Build history of the part. All positions in model axes, mm. A direction names the side the tool comes from. Round coordinates to 2 decimals unless told otherwise and drop trailing zeros. Write each loop counter-clockwise with the first axis right and the second up, starting at its lowest first coordinate (ties: lowest second). Pieces come first, ordered by that corner, then holes. Notation, with made-up numbers: M 74.25,36 L 102.25,36 A18 ccw 102.25,65 Z; hole C 36.5,50 d9. An arc over 180 degrees is marked long. Use a Markdown table: item, result.
from build123d import *

# Parameters (mm, degrees)
F2_W     = 50
F2_H     = 55
F3_DEPTH = 30
F4_W     = 49
F4_H     = 20.1
F5_DEPTH = 50.001
F0_R     = 2.85
F6_DEPTH = 4.9
F0_W     = 7
F0_H     = 6.6
F7_DEPTH = 15
F8_START = 25
F1_W     = 40
F1_H     = 45
F8_DEPTH = 25


# Not quite as in the source:
# - a feature names something its author has since deleted; it is built from what else it names


with BuildPart() as f3:
    # F2 (on Top) → F3 (new body)
    with BuildSketch(Plane.XY):
        with Locations((-48.7460665315, -28.1598071134)):
            Rectangle(F2_W, F2_H)
    extrude(amount=F3_DEPTH)

    # F4 (on face) → F5 (cut, through all)
    with BuildSketch(Plane.YZ.offset(-23.7460665315)):
        with Locations((-27.83, 14.95)):
            Rectangle(F4_W, F4_H)
    extrude(amount=-F5_DEPTH, mode=Mode.SUBTRACT)

    # F0 (on Top) → F6 (cut, through all)
    with BuildSketch(Plane.XY):
        with Locations((-36.0460665315, -28.1598071134)):
            Circle(F0_R)
        with Locations((-61.4460665315, -28.1598071134)):
            Circle(F0_R)
    extrude(amount=F6_DEPTH, mode=Mode.SUBTRACT)

    # F0 (on Top) → F7 (join)
    with BuildSketch(Plane.XY):
        with Locations((-43.6801504195, -28.1598071134)):
            Rectangle(F0_W, F0_H)
    extrude(amount=F7_DEPTH)

    # F1 (on Top) → F8 (cut)
    with BuildSketch(Plane.XY.offset(F8_START)):
        with Locations((-48.7460665315, -27.7248071134)):
            Rectangle(F1_W, F1_H)
    extrude(amount=F8_DEPTH, mode=Mode.SUBTRACT)


solid = f3.part
Q1. Cut at C-C on x = -70. Give the cut face in (y, z), and give its area (3 significant figures).
Response values:
| item | result |
|---|---|
| outline | M -55.66,0 L -0.66,0 L -0.66,30 L -55.66,30 Z; hole M -52.33,4.9 L -3.33,4.9 L -3.33,25 L -52.33,25 Z |
| area | 665 mm2 |
Q2. Cut at D-D on x = -51.5. Give the cut face in (y, z), and give its area (3 significant figures).
Response values:
| item | result |
|---|---|
| outline | M -55.66,0 L -0.66,0 L -0.66,30 L -5.22,30 L -5.22,25 L -3.33,25 L -3.33,4.9 L -52.33,4.9 L -52.33,25 L -50.22,25 L -50.22,30 L -55.66,30 Z |
| area | 440 mm2 |
Q3. Drop flat-ended pins along their axis: P1, Ø2, axis at y = -28, z = 9.5, coming from the +X side; P2, Ø2, axis at x = -44.5, y = -28, coming from the +Z side; P3, Ø5.5, axis at y = -28, z = 9.5, coming from the -X side. Give the stop position or say it passes through.
Response values:
| item | result |
|---|---|
| P1 | stops at x = -40.18 |
| P2 | stops at z = 15 |
| P3 | stops at x = -47.18 |
Q4. Two-plate mould, pull along Y, no slides. Class faces 1 (the flat face through (-27, -28, 30)), 2 (the flat face through (-49, -55.66, 15)), 3 (the flat face through (-44, -28, 15)): +Y half, -Y half, draft (parallel to the pull), parting line (faces both ways), or undercut.
Response values:
| item | result |
|---|---|
| face 1 | draft |
| face 2 | -Y half |
| face 3 | undercut |
Q5. Cut at A-A on y = -18.5. Give the cut face in (x, z), and give its area (3 significant figures).
Response values:
| item | result |
|---|---|
| outline | M -73.75,0 L -23.75,0 L -23.75,4.9 L -73.75,4.9 Z; M -73.75,25 L -68.75,25 L -68.75,30 L -73.75,30 Z; M -28.75,25 L -23.75,25 L -23.75,30 L -28.75,30 Z |
| area | 295 mm2 |
Q6. Which spindle directions (+Z, -Z, +X, -X, +Y, -Y) get a long thin tool onto all of the face, cutting with end or side? Do faces 4 (the flat face through (-28.746, -28, 27)), 5 (the flat face through (-44, -24.86, 10)), 6 (the flat face through (-69, -30, 25)). Say none if no direction does.
Response values:
| item | result |
|---|---|
| face 4 | +Z |
| face 5 | +Z, +X, -X |
| face 6 | +X, -X |
Q7. Drill centre lines: L1, parallel to Z at x = -44, y = -4; L2, parallel to Y at x = -53.5, z = 28.25; L3, parallel to Y at x = -36.5, z = 17. Where is each one in solid material? Low to high.
Response values:
| item | result |
|---|---|
| L1 | z = 0 to 4.9, 25 to 30 |
| L2 | y = -55.66 to -50.22, -5.22 to -0.66 |
| L3 | y = -55.66 to -52.33, -3.33 to -0.66 |
Q8. Cut at B-B on z = 18. Give the cut face in (x, y), and give its area (3 significant figures).
Response values:
| item | result |
|---|---|
| outline | M -73.75,-55.66 L -23.75,-55.66 L -23.75,-52.33 L -73.75,-52.33 Z; M -73.75,-3.33 L -23.75,-3.33 L -23.75,-0.66 L -73.75,-0.66 Z |
| area | 300 mm2 |
